Verification items for the finished model (mm, model axes). Round coordinates to 2 decimals unless told otherwise and drop trailing zeros. Write each loop counter-clockwise with the first axis right and the second up, starting at its lowest first coordinate (ties: lowest second). Pieces come first, ordered by that corner, then holes. Notation, with made-up numbers: (-18.75, 23.25) - (-11.75, 23.25) arc R26 cw to (-11.75, 42.25) - close; hole circle Ø1 at (-26, 56.25). An arc over 180 degrees is marked (long way). Answer as a JSON object with one key per item and string values.
```python
from build123d import *

# Parameters (mm, degrees)
SKETCH1_W           = 55
SKETCH1_H           = 50
BOSS_EXTRUDE1_DEPTH = 3
SKETCH2_R           = 6.35
CUT_EXTRUDE1_DEPTH  = 38.286056375
SKETCH3_R           = 1.5
CUT_EXTRUDE2_DEPTH  = 38.286056375
CIRPATTERN1_COUNT   = 4


with BuildPart() as part:
    # Sketch1 → Boss-Extrude1 (new body)
    with BuildSketch(Plane(origin=(0, 0, 0), x_dir=(1, 0, 0), z_dir=(0, 1, 0))):
        Rectangle(SKETCH1_W, SKETCH1_H)
    extrude(amount=BOSS_EXTRUDE1_DEPTH)

    # Sketch2 → Cut-Extrude1 (cut, through all)
    with BuildSketch(Plane(origin=(0, 3, 0), x_dir=(1, 0, 0), z_dir=(0, 1, 0))):
        with Locations(Location((0, 0, 0), (0, 0, 270))):
            Circle(SKETCH2_R)
    extrude(amount=-CUT_EXTRUDE1_DEPTH, mode=Mode.SUBTRACT)

    # Sketch3 → Cut-Extrude2 (cut, through all)
    with BuildSketch(Plane(origin=(0, 3, 0), x_dir=(1, 0, 0), z_dir=(0, 1, 0))):
        with Locations(Location((-21, 21, 0), (0, 0, 270))):
            Circle(SKETCH3_R)
    cut_extrude2 = extrude(amount=-CUT_EXTRUDE2_DEPTH, mode=Mode.SUBTRACT)

    # CirPattern1: Cut-Extrude2 ×4 about axis
    cirpattern1_axis = Axis((0, 0, 0), (0, 1, 0))
    for i in range(1, CIRPATTERN1_COUNT):
        add(cut_extrude2.rotate(cirpattern1_axis, i * 360 / CIRPATTERN1_COUNT), mode=Mode.SUBTRACT)


solid = part.part
```
Q1. Gauge pin test, flat end, axial feed: P1, Ø2.5, axis at x = -21, z = -21, coming from the -Y side. Record the tip position at first contact, or that the pin passes through.
Geometry check:
{"P1": "passes through"}
Q2. Section check A-A, the plane z = -21. Record the cut outline in (x, y).
Geometry check:
{"outline": "(-27.5, 0) - (-22.5, 0) - (-22.5, 3) - (-27.5, 3) - close; (-19.5, 0) - (19.5, 0) - (19.5, 3) - (-19.5, 3) - close; (22.5, 0) - (27.5, 0) - (27.5, 3) - (22.5, 3) - close"}
Q3. Section check D-D, the plane x = 0. Record the cut outline in (y, z), then the cut area to 3 significant figures.
Geometry check:
{"outline": "(0, -25) - (3, -25) - (3, -6.35) - (0, -6.35) - close; (0, 6.35) - (3, 6.35) - (3, 25) - (0, 25) - close", "area": "112 mm2"}
Q4. Material ranges on line 1 along Z through (x, y) = (21, 2.4); line 2 along X through (y, z) = (1.65, 21); line 3 along Z through (x, y) = (-22, 2.4), recorded low to high. Write a range as [from, to].
Geometry check:
{"line 1": "z = [-25, -22.5], [-19.5, 19.5], [22.5, 25]", "line 2": "x = [-27.5, -22.5], [-19.5, 19.5], [22.5, 27.5]", "line 3": "z = [-25, -22.12], [-19.88, 19.88], [22.12, 25]"}
Q5. Release check for a two-part mould opening along Z. For faces 1 (the cylindrical face through (19.99, 1.52, 22.11)), 2 (the flat face through (0, 1, -25)), 3 (the flat face through (0, 1, 25)), 4 (the flat face through (27.5, 1, 0)) record: released by +Z, released by -Z, zero draft, split by the parting line, or undercut.
Geometry check:
{"face 1": "undercut", "face 2": "released by -Z", "face 3": "released by +Z", "face 4": "zero draft"}
Q6. Section check B-B, the plane y = 0.45. Record the cut outline in (x, z), then the cut area to 3 significant figures.
Geometry check:
{"outline": "(-27.5, -25) - (27.5, -25) - (27.5, 25) - (-27.5, 25) - close; hole circle Ø3 at (-21, -21); hole circle Ø3 at (-21, 21); hole circle Ø12.7 at (0, 0); hole circle Ø3 at (21, -21); hole circle Ø3 at (21, 21)", "area": "2,600 mm2"}
Q7. Section check C-C, the plane x = 21. Record the cut outline in (y, z).
Geometry check:
{"outline": "(0, -25) - (3, -25) - (3, -22.5) - (0, -22.5) - close; (0, -19.5) - (3, -19.5) - (3, 19.5) - (0, 19.5) - close; (0, 22.5) - (3, 22.5) - (3, 25) - (0, 25) - close"}
